Geometry: see drawing. Coordinates: mm, zero at the bounding-box minimum. Coordinates: 2 decimals unless noted, no trailing zeros. Order: outer loops, then holes, each group sorted by start corner. A loop starts at its lowest first (then second) coordinate and runs counter-clockwise, first axis right, second up. Notation, with made-up numbers: M 78.25,24.25 L 122.25,24.25 A20 cw 122.25,54.25 Z; hole C 86.5,-21.75 d8. An arc over 180 degrees is marked long. Answer in a Markdown table with one row per item.
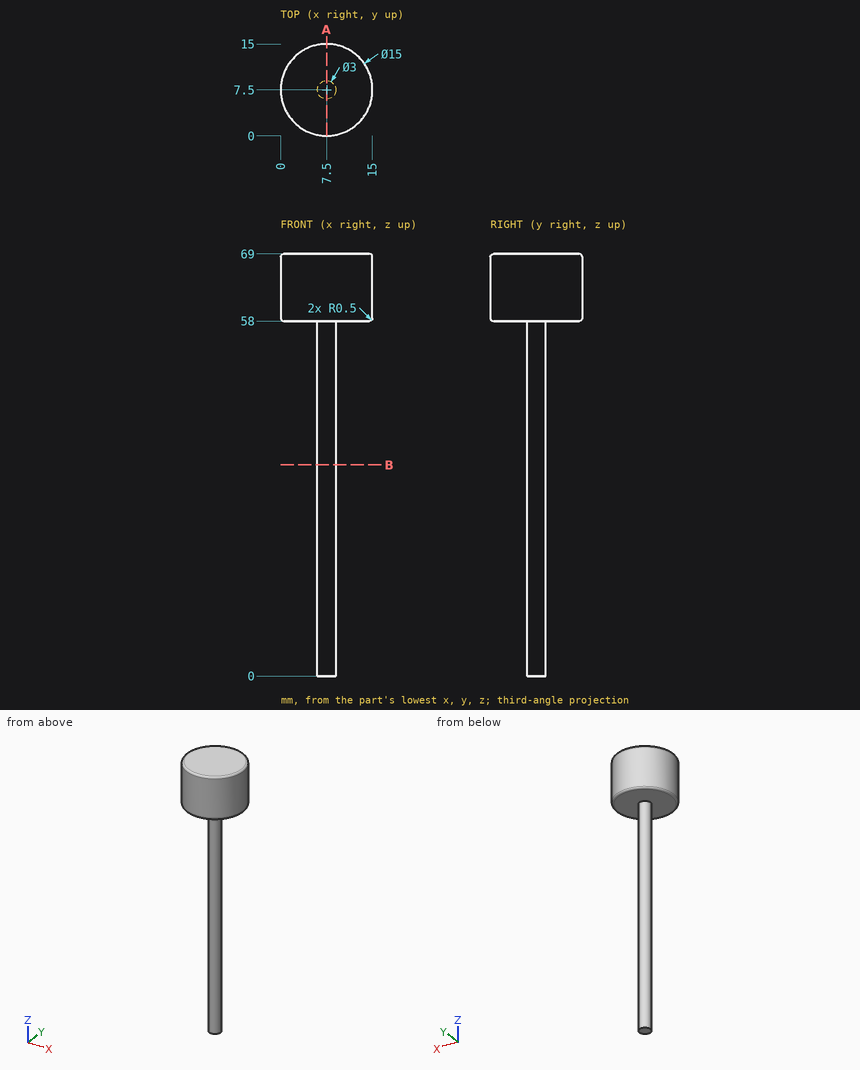
1) Contact query for flat-ended pins moving along their axis: pin 1 (6 mm diameter, centred on y = 6.5, z = 14.5, fed in from +X); pin 2 (1 mm diameter, centred on x = 9, z = 59, fed in from -Y); pin 3 (5 mm diameter, centred on y = 2, z = 31, fed in from +X). Output: stop coordinate, or through.
Resolved:
| item | result |
|---|---|
| pin 1 | stops at x = 9 |
| pin 2 | stops at y = 0.07 |
| pin 3 | passes through |
2) Material intervals for probe 1 along Z at (x, y) = (5.5, 9.5); probe 2 along Y at (x, z) = (8, 21); probe 3 along Y at (x, z) = (6.25, 21), sorted ascending.
Resolved:
| item | result |
|---|---|
| probe 1 | z = 58 to 69 |
| probe 2 | y = 6.09 to 8.91 |
| probe 3 | y = 6.67 to 8.33 |
3) Cut plane B-B, the plane z = 34.5. Output: boundary loops of the cut face in (x, y).
Resolved:
| item | result |
|---|---|
| outline | C 7.5,7.5 d3 |
4) Cut plane A-A, the plane x = 7.5. Output: boundary loops of the cut face in (y, z), and give its area (3 significant figures).
Resolved:
| item | result |
|---|---|
| outline | M 0,58.5 A0.5 ccw 0.5,58 L 6,58 L 6,0 L 9,0 L 9,58 L 14.5,58 A0.5 ccw 15,58.5 L 15,68.5 A0.5 ccw 14.5,69 L 0.5,69 A0.5 ccw 0,68.5 Z |
| area | 339 mm2 |
